Can you work these out from the drawing? Everything is in mm from the part's minimum corner. A direction names the side the tool comes from. Give positions to 0.01 mm unless a question says otherwise; leave off trailing zeros. Loops run counter-clockwise (first coordinate to the right, second up) from the corner with the lowest first, then second, coordinate; pieces in that order, holes last.
Q1. We'd pull the mould along Y, two halves only. Please class the marked faces 4, 5 and 6: +Y half, -Y half, draft (parallel to the pull), parting line (faces both ways), or undercut.
Q2. If we section it at C-C (y = 69.5): Please give me the cut outline in (x, z).
Q3. If we section it at B-B (z = 21): Please give me the cut outline in (x, y).
Q4. If we section it at A-A (y = 29): Please give me the cut outline in (x, z), plus the area to 3 significant figures.
Q5. For the marked faces 1, 2 and 3, which set-ups out of +Z, -Z, +X, -X, +Y, -Y let a thin tool reach every point of the face, with its end or its side?
Q6. I need wall thicknesses on line 1 (Z direction, x = 4, y = 69.05); line 2 (X direction, y = 70, z = 38.5). Which ranges of each line are inside material? Lowest first, please.
Q7. Will these pins go through, and if not, where does the flat tip stop? P1, Ø6, axis at y = 38, z = 44, coming from the -X side; P2, Ø10, axis at x = 13.5, y = 70.5, coming from the +Z side; P3, Ø10, axis at x = 11, y = 57, coming from the +Z side.
Q8. If we section it at D-D (z = 41): Please give me the cut outline in (x, y), plus the area to 3 significant figures.
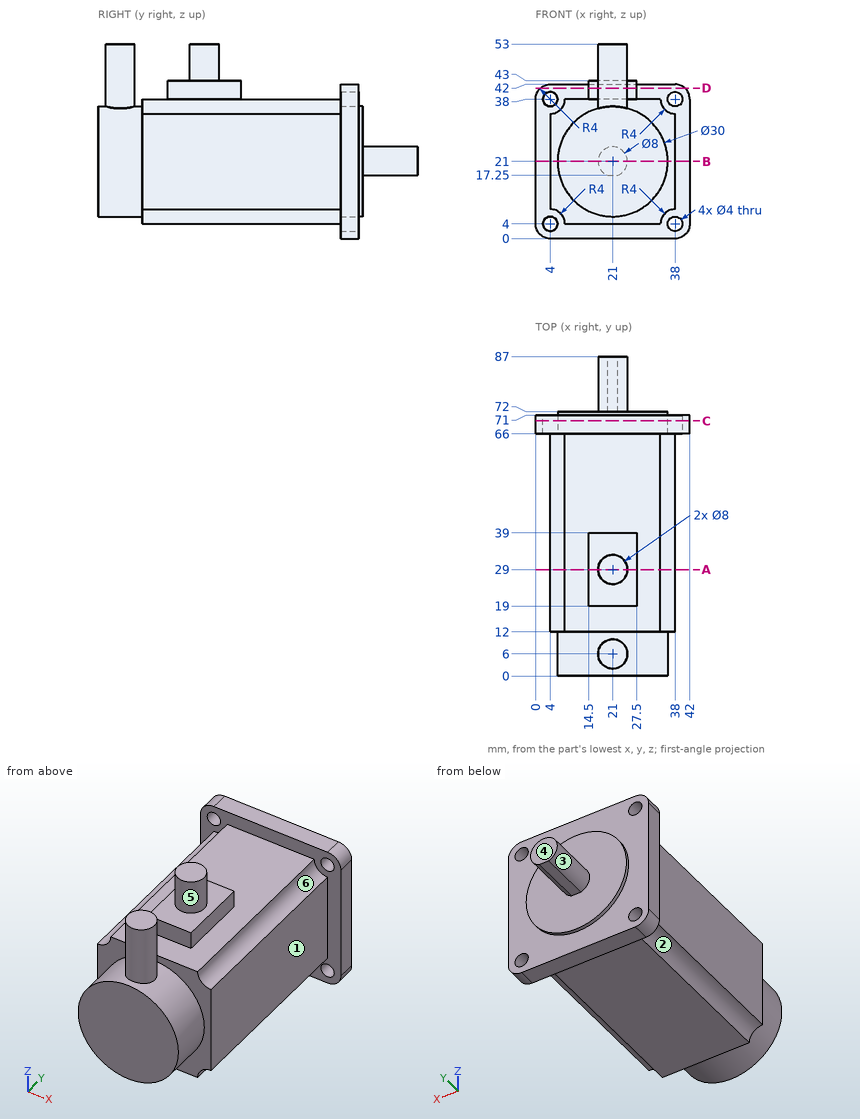
Check sheet entries:
1. face 4: +Y half
1. face 5: undercut
1. face 6: draft
2. outline: (0, 4) arc R4 ccw to (4, 0) - (38, 0) arc R4 ccw to (42, 4) - (42, 38) arc R4 ccw to (38, 42) - (4, 42) arc R4 ccw to (0, 38) - close; hole circle Ø4 at (4, 4); hole circle Ø4 at (4, 38); hole circle Ø4 at (38, 4); hole circle Ø4 at (38, 38)
3. outline: (0, 66) - (4, 66) - (4, 12) - (6, 12) - (6, 0) - (36, 0) - (36, 12) - (38, 12) - (38, 66) - (42, 66) - (42, 71) - (36, 71) - (36, 72) - (25, 72) - (25, 87) - (17, 87) - (17, 72) - (6, 72) - (6, 71) - (0, 71) - close
4. outline: (4, 8) arc R4 cw to (8, 4) - (34, 4) arc R4 cw to (38, 8) - (38, 34) arc R4 cw to (34, 38) - (27.5, 38) - (27.5, 43) - (25, 43) - (25, 53) - (17, 53) - (17, 43) - (14.5, 43) - (14.5, 38) - (8, 38) arc R4 cw to (4, 34) - close
4. area: 1,250 mm2
5. face 1: +Z, -Z, +X, -Y
5. face 2: -Z, -X, -Y
5. face 3: +Y
6. line 1: z = 0 to 2, 6 to 36, 40 to 42
6. line 2: x = 0.03 to 2.06, 5.94 to 36.06, 39.94 to 41.97
7. P1: stops at x = 14.5
7. P2: stops at z = 42
7. P3: stops at z = 38
8. outline: (1.35, 66) - (40.65, 66) - (40.65, 71) - (1.35, 71) - close; (14.5, 19) - (27.5, 19) - (27.5, 39) - (14.5, 39) - close; circle Ø8 at (21, 6)
8. area: 507 mm2
